from build123d import *

# Parameters (mm, degrees)
SKETCH1_W           = 6.35
SKETCH1_H           = 203.2
SKETCH1_H_2         = 29.028571429
BOSS_EXTRUDE1_DEPTH = 6.35
SKETCH2_W           = 6.35
SKETCH2_H           = 203.2
BOSS_EXTRUDE2_DEPTH = 13.56


with BuildPart() as part:
    # Sketch1 → Boss-Extrude1 (new body)
    with BuildSketch(Plane.XY):
        with Locations((-3.175, 0)):
            Rectangle(SKETCH1_W, SKETCH1_H)
        Polygon((6.35, 101.6), (0, 101.6), (0, -101.6), (6.35, -101.6), (6.35, -72.571428571), (6.35, -43.542857143), (6.35, -14.514285714), (6.35, 14.514285714), (6.35, 43.542857143), (6.35, 72.571428571), align=None)
        with Locations((9.525, 87.085714286)):
            Rectangle(SKETCH1_W, SKETCH1_H_2)
        with Locations((9.525, 29.028571429)):
            Rectangle(SKETCH1_W, SKETCH1_H_2)
        with Locations((9.525, -29.028571429)):
            Rectangle(SKETCH1_W, SKETCH1_H_2)
        with Locations((9.525, -87.085714286)):
            Rectangle(SKETCH1_W, SKETCH1_H_2)
    extrude(amount=BOSS_EXTRUDE1_DEPTH)

    # Sketch2 → Boss-Extrude2 (add)
    with BuildSketch(Plane.ZY.offset(6.35)):
        with Locations((3.175, 0)):
            Rectangle(SKETCH2_W, SKETCH2_H)
    extrude(amount=BOSS_EXTRUDE2_DEPTH)


solid = part.part
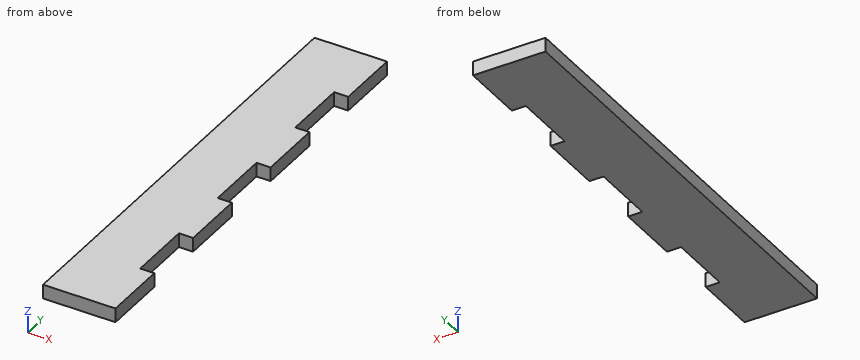
CAD build for the part. Positions are in the model's coordinates, mm. Round coordinates to 2 decimals unless told otherwise and drop trailing zeros. Loops run counter-clockwise (first coordinate to the right, second up) from the corner with the lowest first, then second, coordinate; pieces in that order, holes last. Notation, with made-up numbers: M 20.25,-16 L 56.25,-16 A17 ccw 56.25,16 Z; hole C 56.25,46.25 d4. An arc over 180 degrees is marked long. One line per question, with ' | ' between items. Start each with the question number.
Item 1: Pin check, flat tip, straight feed: pin 1 Ø2 at (y, z) = (-59.5, 1.5) entering from +X. Stop position of the tip, or through.
Item 2: Wall check: line 1 (Y direction, x = 9, z = 4.25); line 2 (X direction, y = -68.5, z = 2.75). Give the ranges that are in metal, low to high.
Item 3: Cut at C-C, the plane y = 50. Write the cut outline in (x, z), plus the area to 3 significant figures.
Item 4: Cut at A-A, the plane x = 11. Write the cut outline in (y, z), plus the area to 3 significant figures.
Item 5: Cut at B-B, the plane z = 5. Write the cut outline in (x, y), plus the area to 3 significant figures.
Responses:
1) pin 1: stops at x = 6.35
2) line 1: y = -101.6 to -72.57, -43.54 to -14.51, 14.51 to 43.54, 72.57 to 101.6 | line 2: x = -19.91 to 6.35
3) outline: M -19.91,0 L 6.35,0 L 6.35,6.35 L -19.91,6.35 Z | area: 167 mm²
4) outline: M -101.6,0 L -72.57,0 L -72.57,6.35 L -101.6,6.35 Z; M -43.54,0 L -14.51,0 L -14.51,6.35 L -43.54,6.35 Z; M 14.51,0 L 43.54,0 L 43.54,6.35 L 14.51,6.35 Z; M 72.57,0 L 101.6,0 L 101.6,6.35 L 72.57,6.35 Z | area: 737 mm²
5) outline: M -19.91,-101.6 L 12.7,-101.6 L 12.7,-72.57 L 6.35,-72.57 L 6.35,-43.54 L 12.7,-43.54 L 12.7,-14.51 L 6.35,-14.51 L 6.35,14.51 L 12.7,14.51 L 12.7,43.54 L 6.35,43.54 L 6.35,72.57 L 12.7,72.57 L 12.7,101.6 L -19.91,101.6 Z | area: 6,070 mm²
